Part model, mm, in its own coordinate system. A direction names the side the tool comes from. Give positions to 0.01 mm unless a question says otherwise; leave off trailing zeros. Order: outer loops, then holes, each group sorted by start corner. A loop starts at its lowest first (then second) coordinate and runs counter-clockwise, first axis right, second up. Notation, with made-up numbers: M -8,44.5 L 6,44.5 A21 cw 6,76.5 Z; hole C 36,9 d8. An arc over 180 degrees is marked long. One line per question, with ' | ' between items.
Autodesk Inventor part; units mm, degrees
ref_plane "YZ Plane" through (0, 0, 0) normal (1, 0, 0) x (0, 1, 0)
ref_plane "XZ Plane" through (0, 0, 0) normal (0, 1, 0) x (-1, 0, 0)
ref_plane "XY Plane" through (0, 0, 0) normal (0, 0, 1) x (1, 0, 0)
sketch "Szkic1" plane through (0, 0, 0) normal (0, 1, 0) x (-1, 0, 0)
  circle A0 centre (0, 0) radius 15
  circle A1 centre (0, 0) radius 40
  circle A2 centre (0, 0) radius 100
  circle A3 centre (0, 0) radius 70
  circle A4 centre (0, 0) radius 65
  line L0 (70, 0) -> (65, 0)
  arc A5 (64.5545, 7.5974) -> (69.7435, 5.9875) centre (67.5065, 7.9448) ccw
  arc A6 (69.7385, -6.0444) -> (64.5482, -7.6502) centre (67.5, -8) ccw
  arc A7 (40.1039, 57.3731) -> (38.8994, 52.0753) centre (40.6782, 54.4567) ccw
  arc A8 (25.6977, 59.7045) -> (29.6864, 63.3933) centre (26.8728, 62.4348) ccw
  arc A9 (-29.6346, 63.4176) -> (-25.6489, 59.7255) centre (-26.8218, 62.4567) ccw
  arc A10 (-38.8568, 52.1071) -> (-40.057, 57.4059) centre (-40.6337, 54.4899) ccw
  arc A11 (-69.7385, 6.0444) -> (-64.5482, 7.6502) centre (-67.5, 8) ccw
  arc A12 (-64.5545, -7.5974) -> (-69.7435, -5.9875) centre (-67.5065, -7.9448) ccw
  arc A13 (-40.1039, -57.3731) -> (-38.8994, -52.0753) centre (-40.6782, -54.4567) ccw
  arc A14 (-25.6977, -59.7045) -> (-29.6864, -63.3933) centre (-26.8728, -62.4348) ccw
  arc A15 (29.6346, -63.4176) -> (25.6489, -59.7255) centre (26.8218, -62.4567) ccw
  arc A16 (38.8568, -52.1071) -> (40.057, -57.4059) centre (40.6337, -54.4899) ccw
  point P0 (-29.6346, 63.4176)
  point P1 (29.6864, 63.3933)
  point P2 (-38.8568, 52.1071)
  point P3 (-69.7385, 6.0444)
  point P4 (-40.1039, -57.3731)
  point P5 (-69.7435, -5.9875)
  point P6 (29.6346, -63.4176)
  point P7 (-29.6864, -63.3933)
  point P8 (38.8568, -52.1071)
  point P9 (40.057, -57.4059)
  point P10 (38.8994, 52.0753)
  point P11 (40.1039, 57.3731)
  dimension "d0" = 30
  dimension "d20" = 200
  dimension "d21" = 140
  dimension "d22" = 130
  dimension "d25" = 10
  dimension "d28" = 360
extrude "Wyciągnięcie proste1" add sketch "Szkic1" along normal blind 1 contours A1 | A2 | L0 A4 A5 A3 | A3 A6 A4 L0 | A4 | A7 A4 A8 A3 | A3 A15 A4 A16 | A9 A4 A10 A3 | A3 A13 A4 A14 | A11 A4 A12 A3
sketch "Szkic3" plane through (0, 1, 0) normal (0, 1, 0) x (1, 0, 0)
  circle A0 centre (0, 0) radius 22.5
  circle A1 centre (-26, 0) radius 2.5
  circle A2 centre (13, -22.5167) radius 2.5
  circle A3 centre (13, 22.5167) radius 2.5
  dimension "d42" = 45
  dimension "d46" = 5
  dimension "d50" = 360
  dimension "d54" = 26
extrude "Wyciągnięcie proste3" cut sketch "Szkic3" against normal blind 10 contours A1 | A2 | A3
sketch "Szkic4" plane through (0, 1, 0) normal (0, 1, 0) x (1, 0, 0)
  point P0 (0, 0)
properties part number "Tarcza_Okładzina" material "Stal, węglowa"
1. Mould opens along X. For faces 3 (the cylindrical face through (-95.38, 0.49, -30.04)), 4 (the cylindrical face through (0.3, 0.5, 65)), 5 (the flat face through (1, 1, -21)) say: released by +X, released by -X, zero draft, split by the parting line, or undercut.
Worked out:
face 3: split by the parting line | face 4: undercut | face 5: zero draft
2. Slice it at C-C on y = 0.3. Give the number of separate pieces and of enclosed holes in the cut face, then the cut area to 3 significant figures.
Worked out:
separate pieces: 1 | enclosed holes: 10 | area: 28,900 mm2
3. Slice it at A-A on z = 0. Give the cut face in (x, y).
Worked out:
outline: M -100,0 L -28.5,0 L -28.5,1 L -100,1 Z; M -23.5,0 L -15,0 L -15,1 L -23.5,1 Z; M 15,0 L 100,0 L 100,1 L 15,1 Z
4. Probe L1, parallel to Z at x = 0, y = 0.3; L2, parallel to Z at x = -50, y = 0.8; L3, parallel to Z at x = 13, y = 0.3. List the from-to ranges inside material, lowest first. Write a range as from..to.
Worked out:
L1: z = -100..-70, -65..-15, 15..65, 70..100 | L2: z = -86.6..-48.99, -41.53..41.53, 48.99..86.6 | L3: z = -99.15..-68.78, -63.69..-25.02, -20.02..-7.48, 7.48..20.02, 25.02..63.69, 68.78..99.15
5. Slice it at B-B on x = 0. Give the cut face in (y, z), then the cut area to 3 significant figures.
Worked out:
outline: M 0,-100 L 1,-100 L 1,-70 L 0,-70 Z; M 0,-65 L 1,-65 L 1,-15 L 0,-15 Z; M 0,15 L 1,15 L 1,65 L 0,65 Z; M 0,70 L 1,70 L 1,100 L 0,100 Z | area: 160 mm2
6. Tool access for faces 1 (the cylindrical face through (60.42, 0.49, -35.35)), 2 (the flat face through (1, 0, -21)): list every direction of +Z, -Z, +X, -X, +Y, -Y with a clear straight run to the whole face (end or side of a thin tool).
Worked out:
face 1: +Y, -Y | face 2: +Z, -Z, +X, -X, -Y
7. Slice it at D-D on z = -41. Give the cut face in (x, y).
Worked out:
outline: M -91.21,0 L -56.74,0 L -56.74,1 L -91.21,1 Z; M -50.44,0 L 50.44,0 L 50.44,1 L -50.44,1 Z; M 56.74,0 L 91.21,0 L 91.21,1 L 56.74,1 Z
